from build123d import *

# Parameters (mm, degrees)
SKETCH_1_R                       = 2.1
SM_BASE_FLANGE_1_DEPTH           = 2
SM_EDGE_FLANGE_1_STRIP_W         = 9.4732
SM_EDGE_FLANGE_1_STRIP_H         = 2
SM_EDGE_FLANGE_1_STRIP_CUT_DEPTH = 37
SM_EDGE_FLANGE_1_DEPTH           = 37
SM_EDGE_FLANGE_1_PROFILE_R       = 2.1
SM_EDGE_FLANGE_1_FLAT_DEPTH      = 2


# Sheet-metal steps are written as plain solids
with BuildPart() as part:
    # Sketch 1 → 基体-法兰1 (new body)
    with BuildSketch(Plane(origin=(0, 0, 0), x_dir=(1, 0, 0), z_dir=(0, 1, 0))):
        with BuildLine():
            Line((-15.5, 16.75), (15.5, 16.75))
            ThreePointArc((15.5, 16.75), (17.621320344, 15.871320344), (18.5, 13.75))
            Line((18.5, 13.75), (18.5, -13.75))
            Line((18.5, -13.75), (-18.5, -13.75))
            Line((-18.5, -13.75), (-18.5, 13.75))
            ThreePointArc((-18.5, 13.75), (-17.621320344, 15.871320344), (-15.5, 16.75))
        make_face()
        with Locations(Location((-10, 6.75, 0), (0, 0, 270))):
            Circle(SKETCH_1_R, mode=Mode.SUBTRACT)
        with Locations(Location((10, 6.75, 0), (0, 0, 90))):
            Circle(SKETCH_1_R, mode=Mode.SUBTRACT)
    extrude(amount=-SM_BASE_FLANGE_1_DEPTH)

    # 边线-法兰1 strip (across the edge) → 边线-法兰1 strip cut (cut)
    with BuildSketch(Plane(origin=(-18.5, 0, 13.75), x_dir=(0, 0, -1), z_dir=(1, 0, 0))):
        with Locations((-2, -1)):
            Rectangle(SM_EDGE_FLANGE_1_STRIP_W, SM_EDGE_FLANGE_1_STRIP_H)
    extrude(amount=SM_EDGE_FLANGE_1_STRIP_CUT_DEPTH, mode=Mode.SUBTRACT)

    # 边线-法兰1 bend section (across the edge) → 边线-法兰1 (add)
    with BuildSketch(Plane(origin=(-18.5, 0, 13.75), x_dir=(0, 0, -1), z_dir=(1, 0, 0))):
        with BuildLine():
            Line((0, 0.7366), (2, 0.7366))
            ThreePointArc((2, 0.7366), (2.215745145, 0.215745145), (2.7366, 0))
            Line((2.7366, 0), (2.7366, -2))
            ThreePointArc((2.7366, -2), (0.801531583, -1.198468417), (0, 0.7366))
        make_face()
    extrude(amount=SM_EDGE_FLANGE_1_DEPTH)

    # 边线-法兰1 profile (on flange) → 边线-法兰1 flat (add)
    with BuildSketch(Plane.XY.offset(13.75)):
        with BuildLine():
            Line((-18.5, 27.5), (-18.5, 0.7366))
            Line((-18.5, 0.7366), (18.5, 0.7366))
            Line((18.5, 0.7366), (18.5, 27.5))
            ThreePointArc((18.5, 27.5), (17.621320344, 29.621320344), (15.5, 30.5))
            Line((15.5, 30.5), (-15.5, 30.5))
            ThreePointArc((-15.5, 30.5), (-17.621320344, 29.621320344), (-18.5, 27.5))
        make_face()
        with Locations((-10, 20.5)):
            Circle(SM_EDGE_FLANGE_1_PROFILE_R, mode=Mode.SUBTRACT)
        with Locations((10, 20.5)):
            Circle(SM_EDGE_FLANGE_1_PROFILE_R, mode=Mode.SUBTRACT)
    extrude(amount=-SM_EDGE_FLANGE_1_FLAT_DEPTH)


solid = part.part
The model under review builds one solid part; all positions refer to its coordinate system, in mm. A direction names the side the tool comes from. Round coordinates to 2 decimals unless told otherwise and drop trailing zeros. Loops run counter-clockwise (first coordinate to the right, second up) from the corner with the lowest first, then second, coordinate; pieces in that order, holes last. Notation, with made-up numbers: M 35.25,-35 L 53.25,-35 A21 cw 53.25,-2 Z; hole C -34.75,89.25 d3. An arc over 180 degrees is marked long. Answer as CSV lines item,"result". Start each with the question number.
Item 1: Consider section A-A (x = -10). Write out the cut boundary in (y, z).
Item 2: Insertion check: P1, Ø3, axis at x = -5.5, z = -3, coming from the +Y side; P2, Ø3, axis at x = -9, y = 2, coming from the -Z side; P3, Ø5.5, axis at x = -10, y = 20.5, coming from the -Z side; P4, Ø2.5, axis at x = 10, z = -6.75, coming from the +Y side. Each pin has a flat end and moves straight along its axis. Give the tip position at first contact, or say it passes through.
Item 3: Mouldability with a two-part tool opening along X and no side actions: class faces 1 (the face through (-17.64, -0.99, -15.85)), 2 (the face through (-11.548, 21.919, 12.764)), 3 (the face through (0, 16, 13.75)) as released by +X, released by -X, zero draft, split by the parting line, or undercut.
Item 4: Consider section B-B (z = -6.75). Write out the cut boundary in (x, y), then the cut area to 3 significant figures.
Item 5: For faces 4 (the face through (-7.918, -0.986, -7.023)), 5 (the face through (0, 0, -3)), list the 3-axis set-ups (+Z, -Z, +X, -X, +Y, -Y) from which the entire face can be reached by the end or side of a thin tool; tool diameter is ignored.
Item 6: Consider section C-C (y = 20.5). Write out the cut boundary in (x, z), then the cut area to 3 significant figures.
Item 7: Consider section D-D (x = -2.5). Write out the cut boundary in (y, z), then the cut area to 3 significant figures.
Item 8: Wall thickness on line 1 (X direction, y = -1.2, z = -6.75); line 2 (Y direction, x = -16.5, z = 0.5); line 3 (Z direction, x = 0, y = 21): over which ranges is each line inside the solid? List them lowest first. Write a range as [from, to].
Answer:
1,outline,"M -2,-16.75 L 0,-16.75 L 0,-8.85 L -2,-8.85 Z; M -2,-4.65 L 0,-4.65 L 0,11.01 A0.74 cw 0.74,11.75 L 18.4,11.75 L 18.4,13.75 L 0.74,13.75 A2.74 ccw -2,11.01 Z; M 22.6,11.75 L 30.5,11.75 L 30.5,13.75 L 22.6,13.75 Z"
2,P1,"stops at y = 0"
2,P2,"stops at z = 11.71"
2,P3,"stops at z = 11.75"
2,P4,"passes through"
3,face 1,"released by -X"
3,face 2,"undercut"
3,face 3,"zero draft"
4,outline,"M -18.5,-2 L -12.1,-2 L -12.1,0 L -18.5,0 Z; M -7.9,-2 L 7.9,-2 L 7.9,0 L -7.9,0 Z; M 12.1,-2 L 18.5,-2 L 18.5,0 L 12.1,0 Z"
4,area,"57.2 mm^2"
5,face 4,"+Y, -Y"
5,face 5,"-Z, +X, -X, +Y"
6,outline,"M -18.5,11.75 L -12.1,11.75 L -12.1,13.75 L -18.5,13.75 Z; M -7.9,11.75 L 7.9,11.75 L 7.9,13.75 L -7.9,13.75 Z; M 12.1,11.75 L 18.5,11.75 L 18.5,13.75 L 12.1,13.75 Z"
6,area,"57.2 mm^2"
7,outline,"M -2,-16.75 L 0,-16.75 L 0,11.01 A0.74 cw 0.74,11.75 L 30.5,11.75 L 30.5,13.75 L 0.74,13.75 A2.74 ccw -2,11.01 Z"
7,area,"121 mm^2"
8,line 1,"x = [-18.5, -12.1], [-7.9, 7.9], [12.1, 18.5]"
8,line 2,"y = [-2, 0]"
8,line 3,"z = [11.75, 13.75]"
